Part print with two shaded views. Sizes in mm from the minimum x, y, z corner. A direction names the side the tool comes from. Coordinates: 2 decimals unless noted, no trailing zeros. Loops run counter-clockwise (first coordinate to the right, second up) from the corner with the lowest first, then second, coordinate; pieces in that order, holes last. Notation, with made-up numbers: (62, 11.25) -> (114, 11.25) arc R8 cw to (114, 19.25) -> close; hole circle Ø9 at (-6, 23). An arc over 180 degrees is marked (long way). Return JSON: item names as keys, results as strings. Group by question number.
(1) Saw through at D-D on x = 2. Write the cut outline in (y, z), then the cut area to 3 significant figures.
(2) Mould opens along X. For the marked faces 1, 2, 3 and 4 say: pulls with the +X half, pulls with the -X half, needs draft (parallel to the pull), parting line crosses it, or undercut.
(3) Probe L1, parallel to Z at x = 5, y = 2; L2, parallel to Y at x = 14, z = 1.3; L3, parallel to Z at x = 7.75, y = 11.5. List the from-to ranges inside material, lowest first.
(4) Saw through at A-A on z = 13. Write the cut outline in (x, y).
(5) Saw through at B-B on z = 24.5. Write the cut outline in (x, y), then the cut area to 3 significant figures.
(6) Saw through at C-C on x = 23. Write the cut outline in (y, z).
(7) Flat gauge pins, fed straight in: pin 1 Ø6 at (x, z) = (12.5, 24.5) entering from +Y; pin 2 Ø3 at (x, y) = (22.5, 19) entering from -Z; pin 3 Ø14 at (x, y) = (9.5, 18.5) entering from +Z; pin 4 Ø6 at (x, z) = (24, 5) entering from +Y. Where does each tip first touch, or does it go through?
(8) Tool access for the marked faces 5 and 6: list every direction of +Z, -Z, +X, -X, +Y, -Y with a clear straight run to the whole face (end or side of a thin tool).
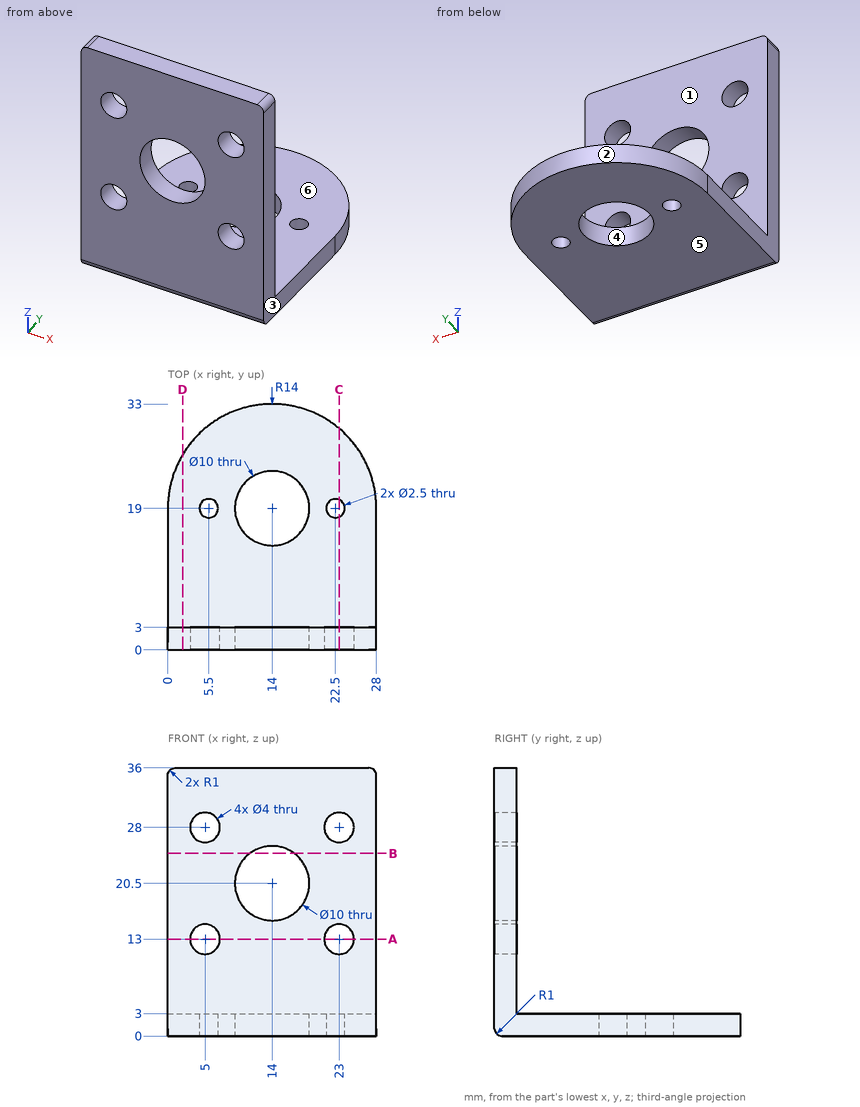
Geometry results:
{
 "1": {"outline": "(0, 1) arc R1 ccw to (1, 0) -> (26.21, 0) -> (26.21, 3) -> (3, 3) -> (3, 36) -> (0, 36) -> close", "area": "177 mm²"},
 "2": {"face 1": "needs draft", "face 2": "parting line crosses it", "face 3": "pulls with the +X half", "face 4": "undercut"},
 "3": {"L1": "0 to 11, 15 to 26, 30 to 36", "L2": "0 to 14, 24 to 33", "L3": "0 to 3"},
 "4": {"outline": "(0, 0) -> (3, 0) -> (3, 3) -> (0, 3) -> close; (7, 0) -> (21, 0) -> (21, 3) -> (7, 3) -> close; (25, 0) -> (28, 0) -> (28, 3) -> (25, 3) -> close"},
 "5": {"outline": "(0, 0) -> (11, 0) -> (11, 3) -> (0, 3) -> close; (17, 0) -> (28, 0) -> (28, 3) -> (17, 3) -> close", "area": "66.0 mm²"},
 "6": {"outline": "(0, 1) arc R1 ccw to (1, 0) -> (17.85, 0) -> (17.85, 3) -> (3, 3) -> (3, 11) -> (0, 11) -> close; (0, 15) -> (3, 15) -> (3, 26) -> (0, 26) -> close; (0, 30) -> (3, 30) -> (3, 36) -> (0, 36) -> close; (20.15, 0) -> (29.72, 0) -> (29.72, 3) -> (20.15, 3) -> close"},
 "7": {"pin 1": "y = 3", "pin 2": "z = 0", "pin 3": "z = 3", "pin 4": "y = 30.65"},
 "8": {"face 5": "-Z, +X, -X, +Y, -Y", "face 6": "+Z, +X, -X, +Y"}
}
